Here's how the part is built. I have some questions about the finished solid (model axes, mm). Face numbers are marked on the shaded views. A direction names the side the tool comes from. Round coordinates to 2 decimals unless told otherwise and drop trailing zeros. Loops run counter-clockwise (first coordinate to the right, second up) from the corner with the lowest first, then second, coordinate; pieces in that order, holes last. Notation, with made-up numbers: (-6, 50) - (51, 50) arc R6 cw to (51, 58) - close; hole circle Ø11 at (64, 38.25). An arc over 180 degrees is marked (long way). Answer as a JSON object with one key per item and string values. Group by question number.
1) I want a section at D-D, the plane x = -1. Please give me the cut outline in (y, z).
2) If I drill on line 1 along Z through (x, y) = (0, -2.5); line 2 along Z through (x, y) = (-1.75, -3.25); line 3 along X through (y, z) = (2.8, 9.7), over which ranges is the centre line in solid material (lowest first)? Write a range as [from, to].
3) I want a section at B-B, the plane z = 0. Please give me the cut outline in (x, y), then the cut area to 3 significant figures.
4) I want a section at A-A, the plane z = -10.3. Please give me the cut outline in (x, y).
5) Which directions (+Z, -Z, +X, -X, +Y, -Y) give clear straight access to the entire face, cutting with the end or side of a thin tool? Please do the marked faces 5 and 6.
6) If we mould it in two halves opening along X, with no side actions, what happens to the marked faces 1, 2, 3 and 4? For each: pulls with the +X half, pulls with the -X half, needs draft (parallel to the pull), parting line crosses it, or undercut.
7) Will these pins go through, and if not, where does the flat tip stop? P1, Ø5, axis at x = -1, z = -10.5, coming from the +Y side; P2, Ø1.5, axis at y = -7, z = 4.5, coming from the +X side.
8) I want a section at C-C, the plane y = -2.25. Please give me the cut outline in (x, z).
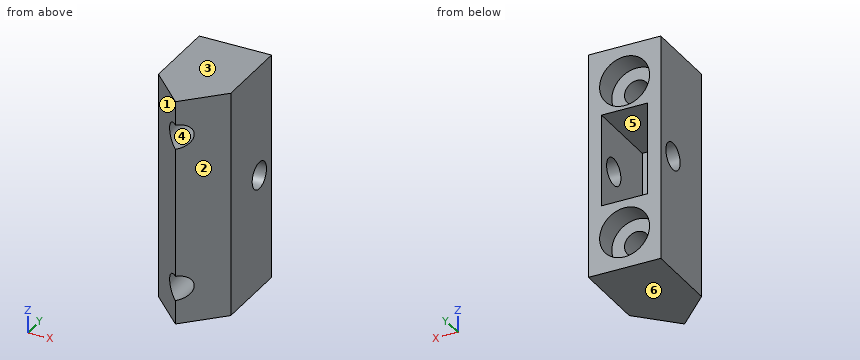
from build123d import *

# Parameters (mm, degrees)
BOSS_EXTRUDE1_DEPTH            = 14.4
BOSS_EXTRUDE1_DEPTH_BACK       = 15
SKETCH2_W                      = 6
SKETCH2_H                      = 12
CUT_EXTRUDE1_DEPTH             = 10
SKETCH3_R                      = 1.75
CUT_EXTRUDE2_DEPTH             = 21.185390757
CBORE_FOR_M3_SHCS1_D           = 3.2
CBORE_FOR_M3_SHCS1_CBORE_D     = 6.5
CBORE_FOR_M3_SHCS1_CBORE_DEPTH = 3


with BuildPart() as part:
    # Sketch1 → Boss-Extrude1 (new, two sides: drawn at the far end of the back side and taken through both)
    with BuildSketch(Plane.XY.offset(-BOSS_EXTRUDE1_DEPTH_BACK)):
        Polygon((-4.7, 5), (4.7, 5), (4.7, -5), (0, -9.7), (-4.7, -5), align=None)
    extrude(amount=BOSS_EXTRUDE1_DEPTH + BOSS_EXTRUDE1_DEPTH_BACK)

    # Sketch2 → Cut-Extrude1 (cut)
    with BuildSketch(Plane(origin=(0, 5, 0), x_dir=(1, 0, 0), z_dir=(0, 1, 0))):
        Rectangle(SKETCH2_W, SKETCH2_H)
    extrude(amount=-CUT_EXTRUDE1_DEPTH, mode=Mode.SUBTRACT)

    # Sketch3 → Cut-Extrude2 (cut, through all)
    with BuildSketch(Plane(origin=(4.7, 0, 0), x_dir=(0, 0, -1), z_dir=(1, 0, 0))):
        with Locations(Location((0, 2, 0), (0, 0, 90))):
            Circle(SKETCH3_R)
    extrude(amount=-CUT_EXTRUDE2_DEPTH, mode=Mode.SUBTRACT)

    # CBORE for M3 SHCS1 (through all)
    with Locations(Plane(origin=(0, 5, 0), x_dir=(1, 0, 0), z_dir=(0, 1, 0))):
        with Locations((0, -9.7), (0, 10.3)):
            CounterBoreHole(CBORE_FOR_M3_SHCS1_D / 2, CBORE_FOR_M3_SHCS1_CBORE_D / 2, CBORE_FOR_M3_SHCS1_CBORE_DEPTH)


solid = part.part
Outcome:
{
 "1": {"outline": "(-8.7, -15) - (5, -15) - (5, -13.39) - (2, -13.39) - (2, -11.55) - (-8.7, -11.55) - close; (-8.7, -9.05) - (2, -9.05) - (2, -7.21) - (5, -7.21) - (5, -6) - (-5, -6) - (-5, 6) - (5, 6) - (5, 6.61) - (2, 6.61) - (2, 8.45) - (-8.7, 8.45) - close; (-8.7, 10.95) - (2, 10.95) - (2, 12.79) - (5, 12.79) - (5, 14.4) - (-8.7, 14.4) - close"},
 "2": {"line 1": "[-15, -11.9], [-8.7, -6], [6, 8.1], [11.3, 14.4]", "line 2": "[-15, -6], [6, 14.4]", "line 3": "[-4.7, -3.25], [3.25, 4.7]"},
 "3": {"outline": "(-4.7, -5) - (0, -9.7) - (4.7, -5) - (4.7, 0.25) - (3, 0.25) - (3, -5) - (-3, -5) - (-3, 0.25) - (-4.7, 0.25) - close; (-4.7, 3.75) - (-3, 3.75) - (-3, 5) - (-4.7, 5) - close; (3, 3.75) - (4.7, 3.75) - (4.7, 5) - (3, 5) - close", "area": "44.2 mm^2"},
 "4": {"outline": "(-4.7, -5) - (-1.6, -8.1) - (-1.6, 2) - (-3.25, 2) - (-3.25, 5) - (-4.7, 5) - close; (1.6, -8.1) - (4.7, -5) - (4.7, 5) - (3.25, 5) - (3.25, 2) - (1.6, 2) - close"},
 "5": {"face 5": "+Y", "face 6": "-Z, +X, -X, +Y, -Y"},
 "6": {"face 1": "pulls with the -X half", "face 2": "pulls with the +X half", "face 3": "needs draft", "face 4": "undercut"},
 "7": {"P1": "y = 5", "P2": "x = 3.45"},
 "8": {"outline": "(-4.7, -15) - (4.7, -15) - (4.7, 14.4) - (-4.7, 14.4) - close; hole (-3, -6) - (3, -6) - (3, 6) - (-3, 6) - close; hole circle Ø3.2 at (0, -10.3); hole circle Ø3.2 at (0, 9.7)"}
}
